Input: part model. Units: mm. Frame: model coordinates. Face numbers are marked on the shaded views. A direction names the side the tool comes from. Coordinates: 2 decimals unless noted, no trailing zeros. Loops run counter-clockwise (first coordinate to the right, second up) from the corner with the lowest first, then second, coordinate; pieces in that order, holes last. Notation, with made-up numbers: (85.25, 6) - (130.25, 6) arc R22 cw to (130.25, 31) - close; hole circle Ø2 at (53, -17.5). An arc over 180 degrees is marked (long way). Write item = value, one per line. Start each with the question number.
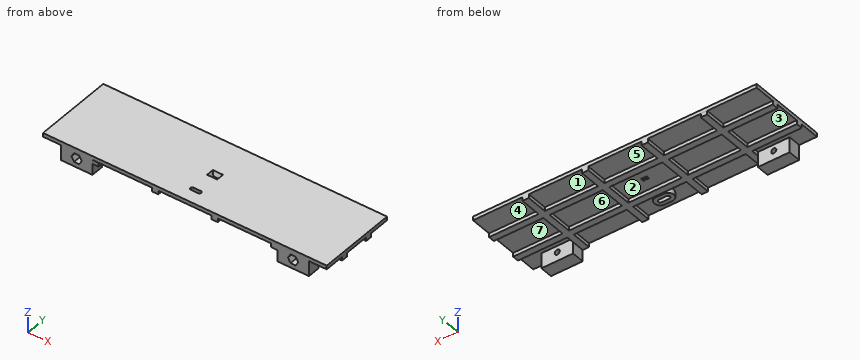
from build123d import *

# Parameters (mm, degrees)
SKETCH_1_W          = 223.7
SKETCH_1_H          = 62.7
EXTRUDE_1_DEPTH     = 3
CUT_EXTRUDE_1_DEPTH = 1
CUT_EXTRUDE_3_DEPTH = 2
EXTRUDE_START       = 4
EXTRUDE_1_2_DEPTH   = 4
SKETCH_13_W         = 25
SKETCH_13_H         = 10
EXTRUDE_2_DEPTH     = 12
SKETCH_14_W         = 41.9
SKETCH_14_H         = 19.999967379
EXTRUDE_3_DEPTH     = 3
SKETCH_15_R         = 2
CUT_EXTRUDE_4_DEPTH = 10
CUT_EXTRUDE_5_DEPTH = 6


with BuildPart() as part:
    # Sketch 1 → Extrude 1 (new body)
    with BuildSketch(Plane.XY):
        Rectangle(SKETCH_1_W, SKETCH_1_H)
    extrude(amount=-EXTRUDE_1_DEPTH)

    # Sketch 2 → Cut-Extrude 1 (cut)
    with BuildSketch(Plane.XY):
        with BuildLine():
            Line((-2.9, -18.55), (2.9, -18.55))
            ThreePointArc((2.9, -18.55), (4.3, -19.95), (2.9, -21.35))
            Line((2.9, -21.35), (-2.9, -21.35))
            ThreePointArc((-2.9, -21.35), (-4.3, -19.95), (-2.9, -18.55))
        make_face()
    extrude(amount=-CUT_EXTRUDE_1_DEPTH, mode=Mode.SUBTRACT)

    # Sketch 5 → Cut-Extrude 3 (cut)
    with BuildSketch(Plane(origin=(0, 0, -3), x_dir=(-1, 0, 0), z_dir=(0, 0, -1))):
        with BuildLine():
            Line((3, -21.55), (-3, -21.55))
            ThreePointArc((-3, -21.55), (-4.6, -19.95), (-3, -18.35))
            Line((-3, -18.35), (3, -18.35))
            ThreePointArc((3, -18.35), (4.6, -19.95), (3, -21.55))
        make_face()
    extrude(amount=-CUT_EXTRUDE_3_DEPTH, mode=Mode.SUBTRACT)

    # Sketch 5_2 → Extrude 1 2 (add)
    with BuildSketch(Plane(origin=(0, 0, -3), x_dir=(-1, 0, 0), z_dir=(0, 0, -1)).offset(EXTRUDE_START)):
        with BuildLine():
            Line((-3, -15.35), (3, -15.35))
            ThreePointArc((3, -15.35), (7.6, -19.95), (3, -24.55))
            Line((3, -24.55), (-3, -24.55))
            ThreePointArc((-3, -24.55), (-7.6, -19.95), (-3, -15.35))
        make_face()
        with BuildLine():
            Line((-3, -18.35), (3, -18.35))
            ThreePointArc((3, -18.35), (4.6, -19.95), (3, -21.55))
            Line((3, -21.55), (-3, -21.55))
            ThreePointArc((-3, -21.55), (-4.6, -19.95), (-3, -18.35))
        make_face(mode=Mode.SUBTRACT)
    extrude(amount=-EXTRUDE_1_2_DEPTH)

    # Sketch 11 → Loft 1 section 0
    with BuildSketch(Plane.XY):
        with BuildLine():
            Line((-4, -3), (4, -3))
            Line((4, -3), (4, 3))
            Line((4, 3), (-4, 3))
            Line((-4, 3), (-4, -3))
        make_face()
    # Sketch 12 → Loft 1 section 1
    with BuildSketch(Plane(origin=(0, 0, -3), x_dir=(-1, 0, 0), z_dir=(0, 0, -1))):
        with BuildLine():
            Line((-2.25, 1.25), (2.25, 1.25))
            Line((2.25, 1.25), (2.25, -1.25))
            Line((2.25, -1.25), (-2.25, -1.25))
            Line((-2.25, -1.25), (-2.25, 1.25))
        make_face()
    loft(mode=Mode.SUBTRACT)

    # Sketch 13 → Extrude 2 (add)
    with BuildSketch(Plane(origin=(0, 0, -3), x_dir=(-1, 0, 0), z_dir=(0, 0, -1))):
        with Locations((85.35, -26.35)):
            Rectangle(SKETCH_13_W, SKETCH_13_H)
        with Locations((-85.35, -26.35)):
            Rectangle(SKETCH_13_W, SKETCH_13_H)
    extrude(amount=EXTRUDE_2_DEPTH)

    # Sketch 14 → Extrude 3 (add)
    with BuildSketch(Plane(origin=(0, 0, -3), x_dir=(-1, 0, 0), z_dir=(0, 0, -1))):
        Polygon((25.95, -15.35), (67.85, -15.35), (67.85, -31.5), (72.85, -31.5), (72.85, -15.35), (111.85, -15.35), (111.85, -10.35), (72.85, -10.35), (72.85, 9.649967379), (111.85, 9.649967379), (111.85, 14.649967379), (72.85, 14.649967379), (72.85, 31.5), (67.85, 31.5), (67.85, 14.649967379), (25.95, 14.649967379), (25.95, 31.35), (20.95, 31.35), (20.95, 14.649967379), (-20.95, 14.649967379), (-20.95, 31.35), (-25.95, 31.35), (-25.95, 14.649967379), (-67.85, 14.649967379), (-67.85, 31.35), (-72.85, 31.35), (-72.85, 14.649967379), (-111.85, 14.649967379), (-111.85, 9.649967379), (-72.85, 9.649967379), (-72.85, -10.35), (-111.82843297, -10.35), (-111.85, -15.35), (-72.85, -15.35), (-72.85, -31.35), (-67.85, -31.35), (-67.85, -15.35), (-25.95, -15.35), (-25.95, -31.35), (-20.95, -31.35), (-20.95, -15.35), (20.95, -15.35), (20.95, -31.35), (25.95, -31.35), align=None)
        with Locations((-46.9, -0.350016311)):
            Rectangle(SKETCH_14_W, SKETCH_14_H, mode=Mode.SUBTRACT)
        with Locations((0, -0.350016311)):
            Rectangle(SKETCH_14_W, SKETCH_14_H, mode=Mode.SUBTRACT)
        with Locations((46.9, -0.350016311)):
            Rectangle(SKETCH_14_W, SKETCH_14_H, mode=Mode.SUBTRACT)
    extrude(amount=EXTRUDE_3_DEPTH)

    # Sketch 15 → Cut-Extrude 4 (cut)
    with BuildSketch(Plane(origin=(0, -31.35, 0), x_dir=(-1, 0, 0), z_dir=(0, -1, 0))):
        with Locations(Location((85.35, 8, 0), (0, 0, 90))):
            Circle(SKETCH_15_R)
        with Locations(Location((-85.35, 8, 0), (0, 0, 90))):
            Circle(SKETCH_15_R)
    extrude(amount=-CUT_EXTRUDE_4_DEPTH, mode=Mode.SUBTRACT)

    # Sketch 16 → Cut-Extrude 5 (cut)
    with BuildSketch(Plane.XZ.offset(31.35)):
        Polygon((-83.329274058, -11.5), (-81.308548116, -8), (-83.329274058, -4.5), (-87.370725942, -4.5), (-89.391451884, -8), (-87.370725942, -11.5), align=None)
        Polygon((87.370725942, -11.5), (89.391451884, -8), (87.370725942, -4.5), (83.329274058, -4.5), (81.308548116, -8), (83.329274058, -11.5), align=None)
    extrude(amount=-CUT_EXTRUDE_5_DEPTH, mode=Mode.SUBTRACT)


solid = part.part
Item 1: Cut plane B-B on x = -46. Return loops of the section in (y, z).
Item 2: Pull-direction query (Y, two-part tool) for the marked faces 1 and 2; classes: pulls with the +Y half, pulls with the -Y half, needs draft (parallel to the pull), parting line crosses it, or undercut.
Item 3: Cut plane A-A on x = 85.35. Return loops of the section in (y, z), plus the area to 3 significant figures.
Item 4: Access query for the marked faces 3, 4, 5, 6 and 7. Directions: +Z, -Z, +X, -X, +Y, -Y. A direction counts if a zero-diameter tool reaches every point of the face in a straight line with its end or side. Return the directions, or none.
Item 5: Ray query, line 1 (X direction, y = 21.5, z = -4); line 2 (X direction, y = -22.6, z = -8); line 3 (Z direction, x = -85, y = -22). Return the intervals inside material, ascending.
Item 6: Pin query (flat end, axial travel): pin 1 (4 mm diameter, centred on x = 65, z = -6.5, fed in from -Y); pin 2 (6.5 mm diameter, centred on x = 0, z = -4.5, fed in from -Y); pin 3 (1.5 mm diameter, centred on y = -17.5, z = -4, fed in from -X). Return the tip coordinate at first contact, or that it passes through.
Recorded:
q1.outline = (-31.35, -3) - (-15.35, -3) - (-15.35, -6) - (-10.35, -6) - (-10.35, -3) - (9.65, -3) - (9.65, -6) - (14.65, -6) - (14.65, -3) - (31.35, -3) - (31.35, 0) - (-31.35, 0) - close
q2.face_1 = needs draft
q2.face_2 = undercut
q3.outline = (-31.35, -15) - (-21.35, -15) - (-21.35, -10) - (-25.35, -10) - (-25.35, -11.5) - (-31.35, -11.5) - close; (-31.35, -4.5) - (-25.35, -4.5) - (-25.35, -6) - (-21.35, -6) - (-21.35, -3) - (-15.35, -3) - (-15.35, -6) - (-10.35, -6) - (-10.35, -3) - (9.65, -3) - (9.65, -6) - (14.65, -6) - (14.65, -3) - (31.35, -3) - (31.35, 0) - (-31.35, 0) - close
q3.area = 280 mm²
q4.face_3 = -Z, -X
q4.face_4 = -Z, +X, +Y
q4.face_5 = -Z, +Y
q4.face_6 = -Z
q4.face_7 = -Z, +X
q5.line_1 = -72.85 to -67.85, -25.95 to -20.95, 20.95 to 25.95, 67.85 to 72.85
q5.line_2 = -97.85 to -87.35, -83.35 to -72.85, 72.85 to 83.35, 87.35 to 97.85
q5.line_3 = -15 to -9.97, -6.03 to 0
q6.pin_1 = -15.35
q6.pin_2 = -31.35
q6.pin_3 = -72.85
